Check sheet for the modelled part. Datum: model origin and axes. Units: mm. Coordinates: 2 decimals unless noted, no trailing zeros. Write each loop counter-clockwise with the first axis right and the second up, starting at its lowest first coordinate (ties: lowest second). Pieces come first, ordered by that corner, then holes. Notation, with made-up numbers: (23, 26) -> (29, 26) arc R27 cw to (29, 62) -> close; hole circle Ø1 at (76.25, 72.5). An arc over 180 degrees is marked (long way). Put each result on its own line as item: value.
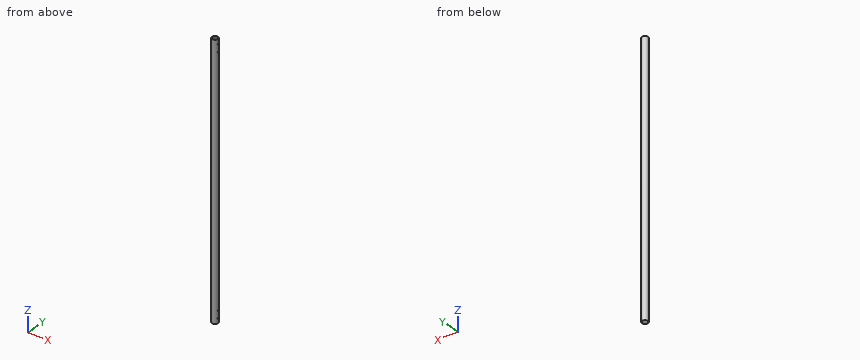
Autodesk Inventor part; units mm, degrees
ref_plane "Work Plane1" through (0, 0, 0) normal (1, 0, 0) x (0, 0, 1)
ref_plane "Work Plane2" through (0, 0, 914.4) normal (0, 0, 1) x (1, 0, 0)
ref_plane "XZ Plane" through (0, 0, 0) normal (0, 1, 0) x (-1, 0, 0)
sketch "Sketch1" plane through (0, 0, 0) normal (0, 0, 1) x (1, 0, 0)
  circle A0 centre (0, 0) radius 21.0312
  circle A1 centre (0, 0) radius 17.4625
  dimension "d0" = 42.0624
  dimension "d1" = 34.925
extrude "Extrusion1" add sketch "Sketch1" along normal blind 1828.8
ref_plane "Work Plane1" through (0, 0, 0) normal (1, 0, 0) x (0, 0, 1)
sketch "Sketch2" plane through (0, 0, 0) normal (1, 0, 0) x (0, 0, 1)
  circle A0 centre (31.75, 0) radius 3.175
  line L0 (-365.76, 0) -> (2194.56, 0)
  line L1 (0, 21.0312) -> (0, -21.0312)
  dimension "d5" = 6.35
  dimension "d6" = 31.75
extrude "Extrusion2" cut sketch "Sketch2" along normal blind 381
pattern_linear "Rectangular Pattern1" count 2 spacing 50.8 along (0, 0, 1) of "Extrusion2"
ref_plane "Work Plane2" through (0, 0, 914.4) normal (0, 0, 1) x (1, 0, 0)
mirror "Mirror1" about plane through (0, 0, 914.4) normal (0, 0, 1) of "Extrusion2", "Rectangular Pattern1"
properties part number "FE-00005-04"
Q1. Depth check by flat-ended pin: P1, Ø2, axis at x = 14.5, z = 310.5, coming from the +Y side; P2, Ø5, axis at x = 7, z = 297, coming from the -Y side; P3, Ø3, axis at y = -2, z = 1605, coming from the +X side; P4, Ø10, axis at x = -6.5, y = -15, coming from the +Z side. Enter the tip coordinate at first touch or a pass-through.
Recorded:
P1: stops at y = 16.13
P2: stops at y = -20.54
P3: stops at x = 21.03
P4: stops at z = 1828.8
Q2. Cross-section at A-A (x = 0). Record the cut outline in (y, z), plus the area to 3 significant figures.
Recorded:
outline: (-21.03, 0) -> (-17.46, 0) -> (-17.46, 1828.8) -> (-21.03, 1828.8) -> close; (17.46, 0) -> (21.03, 0) -> (21.03, 1828.8) -> (17.46, 1828.8) -> close
area: 13,100 mm2
Q3. Material ranges on line 1 along Z through (x, y) = (18.7, 0) (3 decimals); line 2 along Y through (x, z) = (-2.5, 321.5); line 3 along X through (y, z) = (-1.5, 522), recorded low to high.
Recorded:
line 1: z = 0 to 28.575, 34.925 to 79.375, 85.725 to 1743.075, 1749.425 to 1793.875, 1800.225 to 1828.8
line 2: y = -20.88 to -17.28, 17.28 to 20.88
line 3: x = -20.98 to -17.4, 17.4 to 20.98
Q4. Cross-section at B-B (z = 838). Record the cut outline in (x, y) (1 decimal).
Recorded:
outline: circle Ø42.1 at (0, 0); hole circle Ø34.9 at (0, 0)
